Verification items for the finished model (mm, model axes). Face numbers are marked on the shaded views. A direction names the side the tool comes from. Coordinates: 2 decimals unless noted, no trailing zeros. Loops run counter-clockwise (first coordinate to the right, second up) from the corner with the lowest first, then second, coordinate; pieces in that order, holes last. Notation, with made-up numbers: (78, -36) - (88, -36) arc R19 ccw to (88, -26) - close; hole circle Ø11 at (4, 17). An arc over 180 degrees is marked (long way). One line per item, written item: value. Start each with the question number.
(1) Set-up check for the marked faces 1, 2 and 3: record each of +Z, -Z, +X, -X, +Y, -Y from which the full face is reachable in a straight line by a thin tool's end or side.
(2) Section check C-C (z = -7.5). Count the separate pieces of the cut face and the enclosed holes in it, plus the area to 3 significant figures.
(3) Section check A-A (y = -29). Record the boundary of the cut face in (x, z).
(4) Gauge pin test, flat ends, axial feed: P1, Ø2, axis at x = -20.5, z = -3, coming from the -Y side; P2, Ø6.5, axis at y = 29, z = -6, coming from the +X side; P3, Ø1.5, axis at x = -43.5, z = -8, coming from the +Y side. Record the tip position at first contact, or that the pin passes through.
(5) Thickness scan on probe 1 along Y at (x, z) = (-40.75, -6); probe 2 along Y at (x, z) = (-7, -6); probe 3 along Z at (x, y) = (-42.75, 14). Record the ranges inside material, lowest first. Write a range as [from, to].
(6) Section check B-B (x = -45). Record the boundary of the cut face in (y, z), plus the area to 3 significant figures.
```python
from build123d import *

# Parameters (mm, degrees)
SKETCH1_W                    = 52
SKETCH1_H                    = 70
BOSS_EXTRUDE1_DEPTH          = 12
SKETCH2_W                    = 37
SKETCH2_H                    = 14
CUT_EXTRUDE1_DEPTH           = 64.820059542
F_7_0_7_DIAMETER_HOLE1_D     = 7
F_7_0_7_DIAMETER_HOLE1_DEPTH = 60
F_7_0_7_DIAMETER_HOLE1_TIP   = 2.103012167
M6X1_0_TAPPED_HOLE1_D        = 5
M6X1_0_TAPPED_HOLE1_DEPTH    = 18
M6X1_0_TAPPED_HOLE1_TIP      = 1.502151548


with BuildPart() as part:
    # Sketch1 → Boss-Extrude1 (new body)
    with BuildSketch(Plane.XY):
        with Locations((-26, 0)):
            Rectangle(SKETCH1_W, SKETCH1_H)
    extrude(amount=-BOSS_EXTRUDE1_DEPTH)

    # Sketch2 → Cut-Extrude1 (cut, through all)
    with BuildSketch(Plane.XY):
        with Locations((-33.5, 28)):
            Rectangle(SKETCH2_W, SKETCH2_H)
        with Locations((-33.5, -28)):
            Rectangle(SKETCH2_W, SKETCH2_H)
    extrude(amount=-CUT_EXTRUDE1_DEPTH, mode=Mode.SUBTRACT)

    # Ø7.0 (7) Diameter Hole1
    with Locations(Plane.ZY.offset(15)):
        with Locations((-6, 29), (-6, -29)):
            Hole(F_7_0_7_DIAMETER_HOLE1_D / 2, depth=F_7_0_7_DIAMETER_HOLE1_DEPTH)
            with Locations((0, 0, -(F_7_0_7_DIAMETER_HOLE1_DEPTH + F_7_0_7_DIAMETER_HOLE1_TIP / 2))):  # 118° drill point
                Cone(0, F_7_0_7_DIAMETER_HOLE1_D / 2, F_7_0_7_DIAMETER_HOLE1_TIP, mode=Mode.SUBTRACT)

    # M6x1.0 Tapped Hole1
    with Locations(Plane.ZY.offset(52)):
        with Locations((-6, 14), (-6, -14)):
            Hole(M6X1_0_TAPPED_HOLE1_D / 2, depth=M6X1_0_TAPPED_HOLE1_DEPTH)
            with Locations((0, 0, -(M6X1_0_TAPPED_HOLE1_DEPTH + M6X1_0_TAPPED_HOLE1_TIP / 2))):  # 118° drill point
                Cone(0, M6X1_0_TAPPED_HOLE1_D / 2, M6X1_0_TAPPED_HOLE1_TIP, mode=Mode.SUBTRACT)


solid = part.part
```
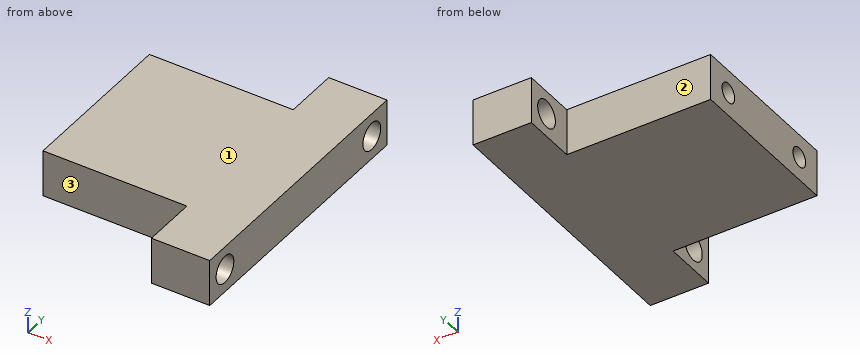
Responses:
1. face 1: +Z, +X, -X, +Y, -Y
1. face 2: +Z, -Z, -X, +Y
1. face 3: +Z, -Z, -X, -Y
2. separate pieces: 3
2. enclosed holes: 0
2. area: 2,270 mm²
3. outline: (-15, -12) - (0, -12) - (0, -9.5) - (-15, -9.5) - close; (-15, -2.5) - (0, -2.5) - (0, 0) - (-15, 0) - close
4. P1: stops at y = -21
4. P2: passes through
4. P3: stops at y = 21
5. probe 1: y = [-21, -16.5], [-11.5, 11.5], [16.5, 21]
5. probe 2: y = [-35, -32.5], [-25.5, 25.5], [32.5, 35]
5. probe 3: z = [-12, -8.5], [-3.5, 0]
6. outline: (-21, -12) - (21, -12) - (21, 0) - (-21, 0) - close; hole circle Ø5 at (-14, -6); hole circle Ø5 at (14, -6)
6. area: 465 mm²
